Build history of the part. All positions in model axes, mm. A direction names the side the tool comes from. Coordinates: 2 decimals unless noted, no trailing zeros. Order: outer loops, then holes, each group sorted by start corner. A loop starts at its lowest first (then second) coordinate and runs counter-clockwise, first axis right, second up. Notation, with made-up numbers: (75.5, 0) - (103.5, 0) arc R16 cw to (103.5, 20) - close; hole circle Ø3 at (84, 77). An arc over 180 degrees is marked (long way). One line per item, written item: value.
from build123d import *

# Parameters (mm, degrees)
F0_R           = 9.525
F1_DEPTH       = 12.7
F2_R           = 6.6675
F3_DEPTH       = 9.525
F4_W           = 1.1938
F4_H           = 2.2352
F6_R           = 14.2875
F6_R_2         = 9.525
F7_DEPTH       = 8.255
F8_R           = 12.827
F9_DEPTH       = 3.81
F10_R          = 10.2235
F11_DEPTH      = 3.81
F12_W          = 0.381
F12_H          = 2.286
F14_R          = 2.6035
F15_DEPTH      = 25.4
F15_DEPTH_BACK = 25.4
F16_SIZE       = 0.508


with BuildPart() as f1:
    # F0 (on Top) → F1 (new body)
    with BuildSketch(Plane.XY):
        Circle(F0_R)
    extrude(amount=F1_DEPTH)

    # F2 (on face) → F3 (cut)
    with BuildSketch(Plane.XY.offset(12.7)):
        Circle(F2_R)
    extrude(amount=-F3_DEPTH, mode=Mode.SUBTRACT)

    # F4 (on Front) → F5 (revolve, cut)
    with BuildSketch(Plane.XZ):
        with Locations((7.2644, 9.9949)):
            Rectangle(F4_W, F4_H)
    revolve(axis=Axis((0, 0, 19.0221574157), (0, 0, 1)), mode=Mode.SUBTRACT)

    # F6 (on face) → F7 (join)
    with BuildSketch(Plane(origin=(0, 0, 0), x_dir=(1, 0, 0), z_dir=(0, 0, -1))):
        Circle(F6_R)
        Circle(F6_R_2, mode=Mode.SUBTRACT)
        Circle(F6_R_2)
    extrude(amount=F7_DEPTH)

    # F8 (on face) → F9 (join)
    with BuildSketch(Plane(origin=(0, 0, -8.255), x_dir=(1, 0, 0), z_dir=(0, 0, -1))):
        Circle(F8_R)
    extrude(amount=F9_DEPTH)

    # F10 (on face) → F11 (cut)
    with BuildSketch(Plane(origin=(0, 0, -12.065), x_dir=(1, 0, 0), z_dir=(0, 0, -1))):
        Circle(F10_R)
    extrude(amount=-F11_DEPTH, mode=Mode.SUBTRACT)

    # F12 (on Front) → F13 (revolve, cut)
    with BuildSketch(Plane.XZ):
        with Locations((12.6365, -9.398)):
            Rectangle(F12_W, F12_H)
    revolve(axis=Axis((0, 0, -8.9314272627), (0, 0, -1)), mode=Mode.SUBTRACT)

    # F14 (on face) → F15 (cut, two sides)
    with BuildSketch(Plane.XY.offset(3.175)) as f15_sk:
        Circle(F14_R)
    extrude(amount=-F15_DEPTH, mode=Mode.SUBTRACT)
    extrude(f15_sk.sketch, amount=F15_DEPTH_BACK, mode=Mode.SUBTRACT)

    # F16
    f16_edges = [f1.edges().sort_by_distance(p)[0] for p in [
        (-10.2235, 0, -12.065),
        (-12.827, 0, -12.065),
    ]]
    chamfer(f16_edges, length=F16_SIZE)


solid = f1.part
1. Probe line 1 along Z through (x, y) = (-4.5, -5.75) (1 decimal); line 2 along Y through (x, z) = (0, -4.5); line 3 along Z through (x, y) = (-1, -4.5) (3 decimals). List the from-to ranges inside material, lowest first.
Values found:
line 1: z = -8.3 to 8.9, 11.1 to 12.7
line 2: y = -14.29 to -2.6, 2.6 to 14.29
line 3: z = -8.255 to 3.175
2. Two-plate mould, pull along Z, no slides. Class faces 6 (the face through (1, -11, -12.065)), 7 (the face through (-2.7, 12.15, -9.38)), 8 (the face through (-0.87, 6.61, 6.07)): pulls with the +Z half, pulls with the -Z half, needs draft (parallel to the pull), parting line crosses it, or undercut.
Values found:
face 6: pulls with the -Z half
face 7: undercut
face 8: needs draft
3. Band-saw the part on A-A, the plane z = -7.75. Give the cut face in (x, y) (1 decimal).
Values found:
outline: circle Ø28.6 at (0, 0); hole circle Ø5.2 at (0, 0)
4. 3-axis set-ups, long thin cutter, end or side, ignore diameter. For faces 1 (the face through (4, -6, 8.877)), 2 (the face through (12.235, -3.853, -11.042)), 3 (the face through (3, 9.3, 0)), 4 (the face through (-2.3, 6.5, 12.7)), 5 (the face through (-14.274, -0.628, -4.07)): which of +Z, -Z, +X, -X, +Y, -Y reach the whole face in a straight line?
Values found:
face 1: none
face 2: -Z
face 3: +Z
face 4: +Z, +X, -X, +Y, -Y
face 5: +Z, -Z
5. Flat gauge pins, fed straight in: P1, Ø4, axis at x = -1, y = 3, coming from the +Z side (3 decimals); P2, Ø5, axis at x = -7, z = -4, coming from the +Y side; P3, Ø1.5, axis at y = -7.5, z = 8, coming from the +X side; P4, Ø3, axis at x = 0, y = 0, coming from the +Z side. Where does each tip first touch, or does it go through?
Values found:
P1: stops at z = 3.175
P2: stops at y = 13.56
P3: stops at x = 6.72
P4: passes through
